Check sheet for the drawn part. Datum: minimum x, y, z corner. Units: mm. Give positions to 0.01 mm unless a question says otherwise; leave off trailing zeros. Loops run counter-clockwise (first coordinate to the right, second up) from the corner with the lowest first, then second, coordinate; pieces in that order, holes last. Notation, with made-up numbers: (-18, 1) - (-10, 1) arc R17 cw to (-10, 29) - close; hole circle Ø10 at (43, 23). An arc over 180 degrees is marked (long way). Answer in a Markdown table with one row per item.
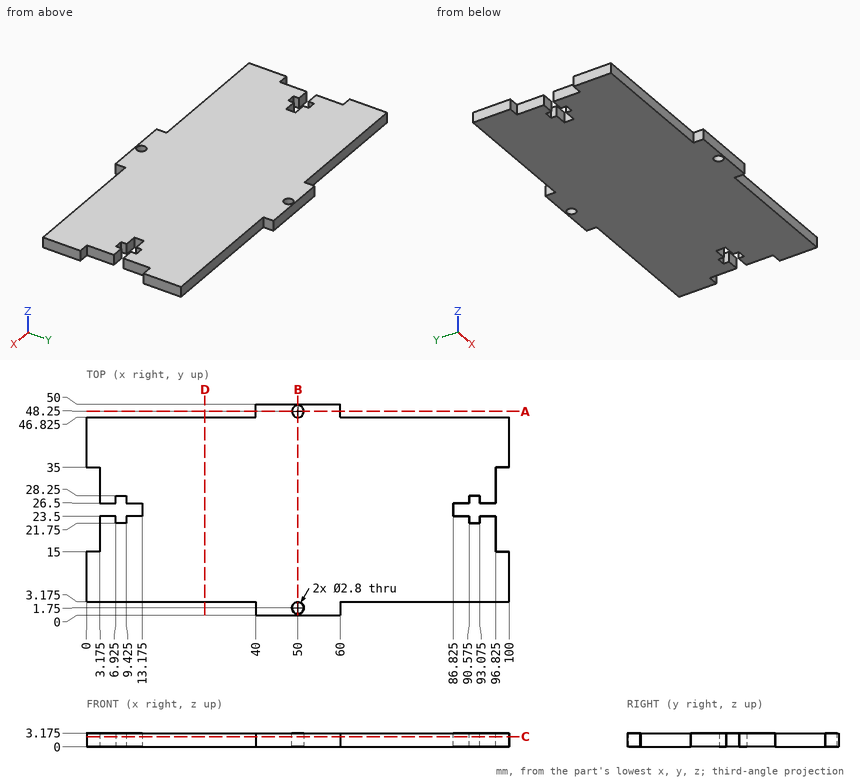
Q1. Thickness scan on line 1 (Y direction, x = 50, z = 1.8); line 2 (Y direction, x = 13, z = 2.2) (3 decimals); line 3 (X direction, y = 1.75, z = 1.95). Record the ranges inside material, lowest first.
Completed:
| item | result |
|---|---|
| line 1 | 0 to 0.35, 3.15 to 46.85, 49.65 to 50 |
| line 2 | 3.175 to 23.5, 26.5 to 46.825 |
| line 3 | 40 to 48.6, 51.4 to 60 |
Q2. Sectioned sample at D-D (x = 28). Record the cut outline in (y, z) (3 decimals).
Completed:
| item | result |
|---|---|
| outline | (3.175, 0) - (46.825, 0) - (46.825, 3.175) - (3.175, 3.175) - close |
Q3. Go/stop test with flat-tipped pins: P1, Ø1.9, axis at y = 23, z = 1, coming from the -X side (3 decimals); P2, Ø1, axis at y = 1.5, z = 2, coming from the +X side; P3, Ø12, axis at x = 55.5, y = 45, coming from the -Z side; P4, Ø1, axis at x = 11, z = 1.5, coming from the +Y side (3 decimals). Record where each tip stops, or that it passes through.
Completed:
| item | result |
|---|---|
| P1 | x = 3.175 |
| P2 | x = 60 |
| P3 | z = 0 |
| P4 | y = 46.825 |
Q4. Sectioned sample at A-A (y = 48.25). Record the cut outline in (x, z) (3 decimals), and give its area (3 significant figures).
Completed:
| item | result |
|---|---|
| outline | (40, 0) - (48.6, 0) - (48.6, 3.175) - (40, 3.175) - close; (51.4, 0) - (60, 0) - (60, 3.175) - (51.4, 3.175) - close |
| area | 54.6 mm^2 |
Q5. Sectioned sample at C-C (z = 2.4). Give the number of separate pieces and of enclosed holes in the cut face, and give its area (3 significant figures).
Completed:
| item | result |
|---|---|
| separate pieces | 1 |
| enclosed holes | 2 |
| area | 4,280 mm^2 |
Q6. Sectioned sample at B-B (x = 50). Record the cut outline in (y, z) (3 decimals).
Completed:
| item | result |
|---|---|
| outline | (0, 0) - (0.35, 0) - (0.35, 3.175) - (0, 3.175) - close; (3.15, 0) - (46.85, 0) - (46.85, 3.175) - (3.15, 3.175) - close; (49.65, 0) - (50, 0) - (50, 3.175) - (49.65, 3.175) - close |
